Read the model definition and answer for the solid it produces. Units are mm, in the model's axes. A direction names the side the tool comes from. Coordinates: 2 decimals unless noted, no trailing zeros. Write each loop counter-clockwise with the first axis right and the second up, starting at its lowest first coordinate (ties: lowest second). Pieces come first, ordered by that corner, then holes. Notation, with made-up numbers: (87.5, 88.25) -> (131.5, 88.25) arc R12 ccw to (131.5, 107.25) -> close; hole circle Ø6 at (-32.5, 86). An arc over 180 degrees is marked (long way). One line per item, written item: value. Start each with the question number.
1. Find section B-B, the plane y = 0. Write down the section's boundary in (x, z), and give its area (3 significant figures).
2. Consider line 1 along Y through (x, z) = (0, 0.45); line 2 along Y through (x, z) = (-6.5, 4.5); line 3 along Z through (x, y) = (-1.25, -23). Determine where each line is inside the solid, lowest interval first.
3. For faces 4 (the flat face through (-7.65, -13, 4)), 5 (the flat face through (2, 0, 1.5)), determine the directions among +Z, -Z, +X, -X, +Y, -Y from which every point of the face is accessible in a straight line to the end or side of a thin tool.
4. Find section C-C, the plane z = 5. Write down the section's boundary in (x, y).
5. Find section A-A, the plane x = -0.5. Write down the section's boundary in (y, z), and give its area (3 significant figures).
6. Given P1, Ø6, axis at x = 1.5, y = 1, coming from the +Z side; P2, Ø4, axis at x = 4, z = 6, coming from the +Y side; P3, Ø0.6, axis at x = 3.5, y = -27.5, coming from the -Z side, each flat-ended and moving along its own axis, determine where each tip first touches the part or whether it passes through.
7. For a pull along Y with two mould halves and no side action, classify faces 1 (the flat face through (0, -13, 7.8)), 2 (the cylindrical face through (-0.17, 1.29, 0.74)), 3 (the cylindrical face through (4.91, 2.643, 0.74)) as pulls with the +Y half, pulls with the -Y half, needs draft (parallel to the pull), parting line crosses it, or undercut.
```python
from build123d import *

# Parameters (mm, degrees)
F0_R     = 1.3
F1_DEPTH = 1.5
F0_W     = 15.3
F0_H     = 20.2
F2_DEPTH = 7.8
F3_W     = 0.5
F3_H     = 0.4
F4_DEPTH = 8


with BuildPart() as f1:
    # F0 (on Top) → F1 (new body)
    with BuildSketch(Plane.XY):
        with BuildLine():
            Line((-5.272679, 2.234062), (-7.65, -2.7))
            Line((-7.65, -2.7), (7.65, -2.7))
            Line((7.65, -2.7), (5.272679, 2.234062))
            ThreePointArc((5.272679, 2.234062), (4.903745, 2.646777), (4.371796, 2.8))
            Line((4.371796, 2.8), (-4.371796, 2.8))
            ThreePointArc((-4.371796, 2.8), (-4.903745, 2.646777), (-5.272679, 2.234062))
        make_face()
        Circle(F0_R, mode=Mode.SUBTRACT)
    extrude(amount=F1_DEPTH)

    # F0 (on Top) → F2 (join)
    with BuildSketch(Plane.XY):
        with Locations((0, -12.8)):
            Rectangle(F0_W, F0_H)
    extrude(amount=F2_DEPTH)

    # F3 (on face) → F4 (join)
    with BuildSketch(Plane.XZ.offset(22.9)):
        with Locations((-3.75, 2.8)):
            Rectangle(F3_W, F3_H)
        with Locations((-1.25, 2.8)):
            Rectangle(F3_W, F3_H)
        with Locations((1.25, 2.8)):
            Rectangle(F3_W, F3_H)
        with Locations((3.75, 2.8)):
            Rectangle(F3_W, F3_H)
    extrude(amount=F4_DEPTH)


solid = f1.part
```
Answer block:
1. outline: (-6.35, 0) -> (-1.3, 0) -> (-1.3, 1.5) -> (-6.35, 1.5) -> close; (1.3, 0) -> (6.35, 0) -> (6.35, 1.5) -> (1.3, 1.5) -> close
1. area: 15.1 mm2
2. line 1: y = -22.9 to -1.3, 1.3 to 2.8
2. line 2: y = -22.9 to -2.7
2. line 3: z = 2.6 to 3
3. face 4: +Z, -Z, -X, +Y, -Y
3. face 5: +Z, +X, -X, +Y
4. outline: (-7.65, -22.9) -> (7.65, -22.9) -> (7.65, -2.7) -> (-7.65, -2.7) -> close
5. outline: (-22.9, 0) -> (-1.2, 0) -> (-1.2, 1.5) -> (-2.7, 1.5) -> (-2.7, 7.8) -> (-22.9, 7.8) -> close; (1.2, 0) -> (2.8, 0) -> (2.8, 1.5) -> (1.2, 1.5) -> close
5. area: 162 mm2
6. P1: stops at z = 1.5
6. P2: stops at y = -2.7
6. P3: stops at z = 2.6
7. face 1: needs draft
7. face 2: undercut
7. face 3: pulls with the +Y half
